Geometry: final body of the model. Coordinates: model frame, mm. Face numbers are marked on the shaded views. Give positions to 0.01 mm unless a question says otherwise; leave off trailing zeros. Order: outer loops, then holes, each group sorted by start corner. A loop starts at its lowest first (then second) coordinate and runs counter-clockwise, first axis right, second up. Notation, with made-up numbers: (40.25, 24.25) -> (61.25, 24.25) arc R13 cw to (61.25, 47.25) -> close; hole circle Ø3 at (-34, 60.5). An arc over 180 degrees is marked (long way). One line per question, with ' | ' between items. Start each with the question number.
(1) Section A-A (z = -1.25). State how many separate pieces and enclosed holes the cut face has, then the cut area to 3 significant figures.
(2) Section B-B (x = 0.75). Return loops of the section in (y, z).
(3) Section C-C (x = -2.75). Return loops of the section in (y, z).
(4) Mould query, pull axis Y, two halves, no side actions, for the marked faces 1, 2 and 3. Classes: +Y half, -Y half, draft (parallel to the pull), parting line (faces both ways), or undercut.
(5) Section D-D (y = 0.5). Return loops of the section in (x, z), then the cut area to 3 significant figures.
(6) Ray query, L1, parallel to Y at x = 0, z = -1.5; L2, parallel to X at y = -27.94, z = 2.5; L3, parallel to Y at x = -2.75, z = -4. Return the intervals inside material, ascending.
(7) First-contact query: pin 1 Ø1 at (x, z) = (-5.5, -3.5) entering from +Y; pin 2 Ø5 at (y, z) = (-2.5, 3) entering from -X; pin 3 Ø9 at (x, y) = (0, 27.94) entering from +Z; pin 4 Ø1.5 at (y, z) = (2, -3.5) entering from +X. Flat tips, straight axial feed; report the tip coordinate or a pass-through.
```python
from build123d import *

# Parameters (mm, degrees)
SKETCH1_W          = 16
SKETCH1_H          = 71.6
BODY_DEPTH         = 5
SKETCH2_R          = 4
TOP_HOLE_DEPTH     = 39.021572824
CUT_EXTRUDE1_DEPTH = 39.021572824
FILLET1_R          = 8


with BuildPart() as part:
    # Sketch1 → Body (new, symmetric)
    with BuildSketch(Plane.XY):
        Rectangle(SKETCH1_W, SKETCH1_H)
    extrude(amount=BODY_DEPTH, both=True)

    # Sketch2 → Top Hole (cut, through all)
    with BuildSketch(Plane.XY.offset(5)):
        with Locations((0, 27.94)):
            Circle(SKETCH2_R)
    top_hole = extrude(amount=-TOP_HOLE_DEPTH, mode=Mode.SUBTRACT)

    # Bottom Hole: Top Hole across plane
    add(top_hole.mirror(Plane.ZX), mode=Mode.SUBTRACT)

    # Sketch3 → Cut-Extrude1 (cut, symmetric)
    with BuildSketch(Plane.XY.offset(5)):
        with BuildLine():
            Line((-8, 17.94), (-8, -17.94))
            ThreePointArc((-8, -17.94), (-5.626994529, 0), (-8, 17.94))
        make_face()
    cut_extrude1 = extrude(amount=CUT_EXTRUDE1_DEPTH, both=True, mode=Mode.SUBTRACT)

    # Mirror1: Cut-Extrude1 across plane
    add(cut_extrude1.mirror(Plane(origin=(0, 0, 0), x_dir=(0, 0, 1), z_dir=(1, 0, 0))), mode=Mode.SUBTRACT)

    # Fillet1
    fillet1_edges = [part.edges().sort_by_distance(p)[0] for p in [
        (8, -35.8, 0),
        (-8, -35.8, 0),
        (8, 35.8, 0),
        (-8, 35.8, 0),
        (-8, 17.94, 0),
        (-8, -17.94, 0),
        (8, -17.94, 0),
        (8, 17.94, 0),
    ]]
    fillet(fillet1_edges, radius=FILLET1_R - 0.0001)  # a hair under: the kernel refuses the full size


solid = part.part
```
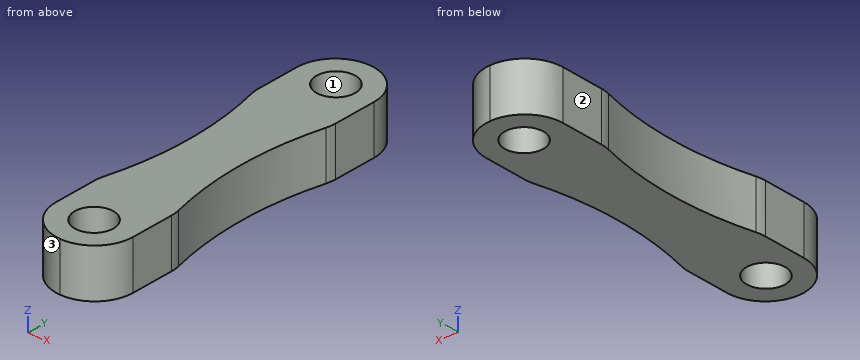
Response:
1) separate pieces: 1 | enclosed holes: 2 | area: 876 mm^2
2) outline: (-35.76, -5) -> (-31.87, -5) -> (-31.87, 5) -> (-35.76, 5) -> close; (-24.01, -5) -> (24.01, -5) -> (24.01, 5) -> (-24.01, 5) -> close; (31.87, -5) -> (35.76, -5) -> (35.76, 5) -> (31.87, 5) -> close
3) outline: (-35.31, -5) -> (-30.84, -5) -> (-30.84, 5) -> (-35.31, 5) -> close; (-25.04, -5) -> (25.04, -5) -> (25.04, 5) -> (-25.04, 5) -> close; (30.84, -5) -> (35.31, -5) -> (35.31, 5) -> (30.84, 5) -> close
4) face 1: undercut | face 2: draft | face 3: -Y half
5) outline: (-5.63, -5) -> (5.63, -5) -> (5.63, 5) -> (-5.63, 5) -> close | area: 113 mm^2
6) L1: y = -35.8 to -31.94, -23.94 to 23.94, 31.94 to 35.8 | L2: x = -8 to -4, 4 to 8 | L3: y = -35.31 to -30.84, -25.04 to 25.04, 30.84 to 35.31
7) pin 1: stops at y = 34.05 | pin 2: stops at x = -5.81 | pin 3: stops at z = 5 | pin 4: stops at x = 5.68
